Here's how the part is built. I have some questions about the finished solid (model axes, mm). A direction names the side the tool comes from. Round coordinates to 2 decimals unless told otherwise and drop trailing zeros. Order: outer loops, then holes, each group sorted by start corner. A loop starts at its lowest first (then second) coordinate and runs counter-clockwise, first axis right, second up.
```python
from build123d import *

# Parameters (mm, degrees)
SKETCH1_W           = 51
SKETCH1_H           = 64
BOSS_EXTRUDE1_DEPTH = 3.1
SKETCH2_R           = 1.2
CUT_EXTRUDE1_DEPTH  = 3.1
BOSS_EXTRUDE2_DEPTH = 5.4
SKETCH4_W           = 8.5
SKETCH4_H           = 7.5
BOSS_EXTRUDE4_DEPTH = 2.5


with BuildPart() as part:
    # Sketch1 → Boss-Extrude1 (new body)
    with BuildSketch(Plane(origin=(0, 0, 0), x_dir=(1, 0, 0), z_dir=(0, 1, 0))):
        Rectangle(SKETCH1_W, SKETCH1_H)
    extrude(amount=BOSS_EXTRUDE1_DEPTH)

    # Sketch2 → Cut-Extrude1 (cut)
    with BuildSketch(Plane(origin=(0, 3.1, 0), x_dir=(1, 0, 0), z_dir=(0, 1, 0))):
        with Locations((-23, 29.5)):
            Circle(SKETCH2_R)
        with Locations((23, 29.5)):
            Circle(SKETCH2_R)
        with Locations((23, -29.5)):
            Circle(SKETCH2_R)
        with Locations((-23, -29.5)):
            Circle(SKETCH2_R)
    extrude(amount=-CUT_EXTRUDE1_DEPTH, mode=Mode.SUBTRACT)

    # Sketch3 → Boss-Extrude2 (add)
    with BuildSketch(Plane(origin=(0, 3.1, 0), x_dir=(1, 0, 0), z_dir=(0, 1, 0))):
        with BuildLine():
            Line((-19, 28), (19, 28))
            ThreePointArc((19, 28), (21.828427125, 26.828427125), (23, 24))
            Line((23, 24), (23, -24))
            ThreePointArc((23, -24), (21.828427125, -26.828427125), (19, -28))
            Line((19, -28), (-19, -28))
            ThreePointArc((-19, -28), (-21.828427125, -26.828427125), (-23, -24))
            Line((-23, -24), (-23, 24))
            ThreePointArc((-23, 24), (-21.828427125, 26.828427125), (-19, 28))
        make_face()
    extrude(amount=BOSS_EXTRUDE2_DEPTH)

    # Sketch4 → Boss-Extrude4 (add)
    with BuildSketch(Plane(origin=(0, 8.5, 0), x_dir=(1, 0, 0), z_dir=(0, 1, 0))):
        with Locations((-14, 20.5)):
            Rectangle(SKETCH4_W, SKETCH4_H)
        with Locations((0, 20.5)):
            Rectangle(SKETCH4_W, SKETCH4_H)
        with Locations((14, 20.5)):
            Rectangle(SKETCH4_W, SKETCH4_H)
        Polygon((9.75, 11.25), (9.75, 3.75), (18.25, 3.75), (18.25, 11.25), (14, 11.25), align=None)
        with Locations((0, 7.5)):
            Rectangle(SKETCH4_W, SKETCH4_H)
        with Locations((-14, 7.5)):
            Rectangle(SKETCH4_W, SKETCH4_H)
        Polygon((-18.25, -1.75), (-18.25, -5.5), (-18.25, -9.25), (-9.75, -9.25), (-9.75, -1.75), align=None)
        with Locations((0, -5.5)):
            Rectangle(SKETCH4_W, SKETCH4_H)
        Polygon((18.25, -9.25), (18.25, -5.5), (18.25, -1.75), (9.75, -1.75), (9.75, -9.25), align=None)
        with Locations((14, -18.5)):
            Rectangle(SKETCH4_W, SKETCH4_H)
        with Locations((0, -18.5)):
            Rectangle(SKETCH4_W, SKETCH4_H)
        with Locations((-14, -18.5)):
            Rectangle(SKETCH4_W, SKETCH4_H)
    extrude(amount=BOSS_EXTRUDE4_DEPTH)


solid = part.part
```
1. If we section it at D-D, the plane x = -21: Write out the boundary of the cut face in (y, z), and give its area (3 significant figures).
Evaluation:
outline: (0, -32) - (3.1, -32) - (3.1, -27.46) - (8.5, -27.46) - (8.5, 27.46) - (3.1, 27.46) - (3.1, 32) - (0, 32) - close
area: 495 mm2
2. On a 3-axis mill with a long thin cutter (end or side, diameter ignored), from which of +Z, -Z, +X, -X, +Y, -Y can I reach the whole of each face in a straight line? I mean faces 1 (the flat face through (-14, 10, -11.25)), 2 (the flat face through (-18.25, 10, -7)), 3 (the flat face through (4.25, 10, 19)), 4 (the cylindrical face through (21.859, 5.762, 26.797)), 5 (the flat face through (-14, 10, 22.25)). Say none if no direction works.
Evaluation:
face 1: +X, -X, +Y
face 2: +Z, -Z, -X, +Y
face 3: +Z, -Z, +Y
face 4: +Z, +X, +Y
face 5: +Z, +X, -X, +Y
3. I need wall thicknesses on probe 1 along Z at (x, y) = (-15.5, 9); probe 2 along Z at (x, y) = (-23, 1.5); probe 3 along X at (y, z) = (2.1, -29.5). Which ranges of each line are inside material? Lowest first, please.
Evaluation:
probe 1: z = -24.25 to -16.75, -11.25 to -3.75, 1.75 to 9.25, 14.75 to 22.25
probe 2: z = -32 to -30.7, -28.3 to 28.3, 30.7 to 32
probe 3: x = -25.5 to -24.2, -21.8 to 21.8, 24.2 to 25.5
4. If we section it at B-B, the plane y = 7.75: Write out the boundary of the cut face in (x, z), and give its area (3 significant figures).
Evaluation:
outline: (-23, -24) arc R4 ccw to (-19, -28) - (19, -28) arc R4 ccw to (23, -24) - (23, 24) arc R4 ccw to (19, 28) - (-19, 28) arc R4 ccw to (-23, 24) - close
area: 2,560 mm2
5. If we section it at C-C, the plane z = 21.5: Write out the boundary of the cut face in (x, y).
Evaluation:
outline: (-25.5, 0) - (25.5, 0) - (25.5, 3.1) - (23, 3.1) - (23, 8.5) - (18.25, 8.5) - (18.25, 11) - (9.75, 11) - (9.75, 8.5) - (4.25, 8.5) - (4.25, 11) - (-4.25, 11) - (-4.25, 8.5) - (-9.75, 8.5) - (-9.75, 11) - (-18.25, 11) - (-18.25, 8.5) - (-23, 8.5) - (-23, 3.1) - (-25.5, 3.1) - close
6. If we mould it in two halves opening along X, with no side actions, what happens to faces 6 (the flat face through (-23, 6, 0)), 7 (the flat face through (18.25, 10, -20)), 8 (the flat face through (9.75, 10, -8)), 9 (the flat face through (0, 10, 9.25))? For each: released by +X, released by -X, zero draft, split by the parting line, or undercut.
Evaluation:
face 6: released by -X
face 7: released by +X
face 8: undercut
face 9: zero draft
7. I'm going to push flat-ended pins straight in: P1, Ø4, axis at y = 8, z = -21.5, coming from the -X side; P2, Ø1.2, axis at y = 9.5, z = 5, coming from the -X side; P3, Ø2, axis at x = -23, z = -29.5, coming from the +Y side; P4, Ø1.2, axis at x = 0, y = 9.5, coming from the +Z side. Where does each tip first touch, or does it pass through?
Evaluation:
P1: stops at x = -23
P2: stops at x = -18.25
P3: passes through
P4: stops at z = 22.25
8. If we section it at A-A, the plane z = -29.5: Write out the boundary of the cut face in (x, y), and give its area (3 significant figures).
Evaluation:
outline: (-25.5, 0) - (-24.2, 0) - (-24.2, 3.1) - (-25.5, 3.1) - close; (-21.8, 0) - (21.8, 0) - (21.8, 3.1) - (-21.8, 3.1) - close; (24.2, 0) - (25.5, 0) - (25.5, 3.1) - (24.2, 3.1) - close
area: 143 mm2
